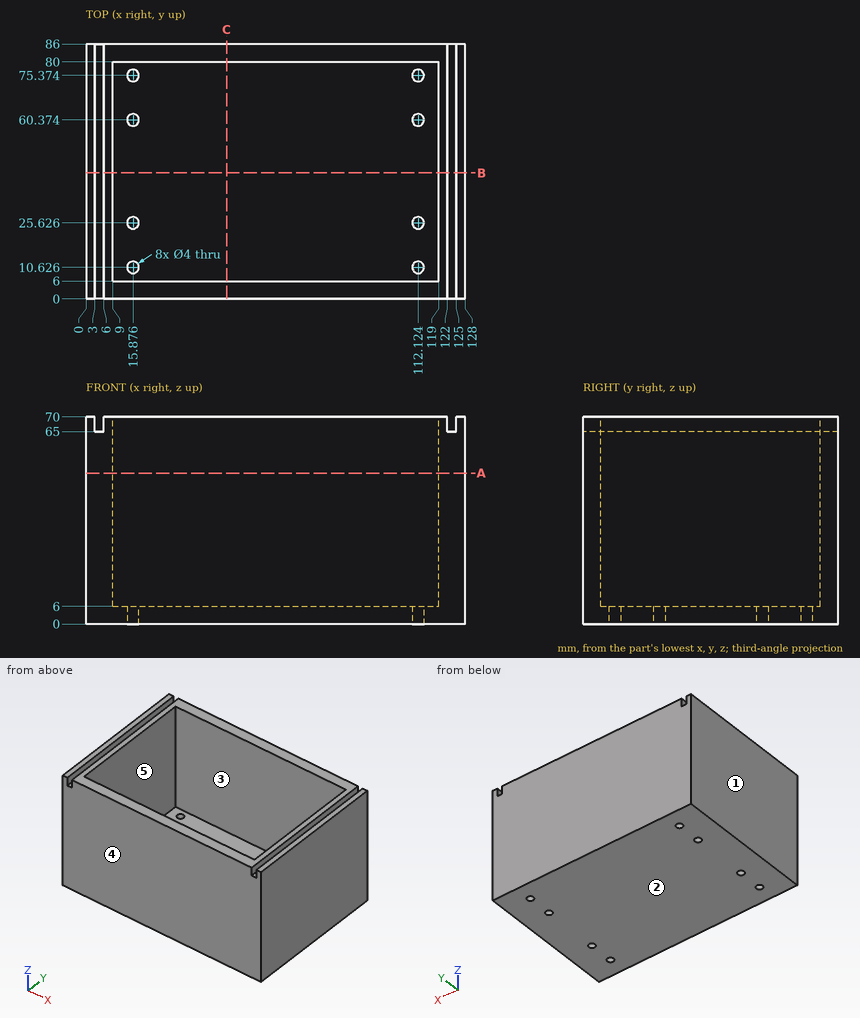
Part print with two shaded views. Sizes in mm from the minimum x, y, z corner. A direction names the side the tool comes from. Coordinates: 2 decimals unless noted, no trailing zeros. Write each loop counter-clockwise with the first axis right and the second up, starting at its lowest first coordinate (ties: lowest second). Pieces come first, ordered by that corner, then holes. Notation, with made-up numbers: (-27, -26) - (-6, -26) arc R19 ccw to (-6, -13) - close; hole circle Ø3 at (-12, -20.5). An arc over 180 degrees is marked (long way). One line per item, written item: value. Start each with the question number.
1. Slice it at B-B (y = 42.5). Write the cut outline in (x, z), plus the area to 3 significant figures.
2. Tool access for the marked faces 4 and 5: list every direction of +Z, -Z, +X, -X, +Y, -Y with a clear straight run to the whole face (end or side of a thin tool).
3. Slice it at C-C (x = 47.5). Write the cut outline in (y, z).
4. Probe line 1 (Y direction, x = 75, z = 52.5); line 2 (X direction, y = 79.5, z = 45.5); line 3 (Z direction, x = 44.5, y = 78.5). List the from-to ranges inside material, lowest first. Write a range as from..to.
5. Slice it at A-A (z = 51). Write the cut outline in (x, y).
6. Flat gauge pins, fed straight in: pin 1 (1 mm diameter, centred on x = 24, y = 16, fed in from +Z); pin 2 (6 mm diameter, centred on x = 19.5, y = 15.5, fed in from -Z); pin 3 (0.9 mm diameter, centred on x = 124, y = 52.5, fed in from +Z); pin 4 (2.5 mm diameter, centred on x = 112.12, y = 10.63, fed in from -Z). Where does each tip first touch, or does it go through?
7. Mould opens along X. For the marked faces 1, 2 and 3 say: released by +X, released by -X, zero draft, split by the parting line, or undercut.
Answers below:
1. outline: (0, 0) - (128, 0) - (128, 70) - (125, 70) - (125, 65) - (122, 65) - (122, 70) - (119, 70) - (119, 6) - (9, 6) - (9, 70) - (6, 70) - (6, 65) - (3, 65) - (3, 70) - (0, 70) - close
1. area: 1,890 mm^2
2. face 4: +Z, -Z, +X, -X, -Y
2. face 5: +Z
3. outline: (0, 0) - (86, 0) - (86, 70) - (80, 70) - (80, 6) - (6, 6) - (6, 70) - (0, 70) - close
4. line 1: y = 0..6, 80..86
4. line 2: x = 0..9, 119..128
4. line 3: z = 0..6
5. outline: (0, 0) - (128, 0) - (128, 86) - (0, 86) - close; hole (9, 6) - (119, 6) - (119, 80) - (9, 80) - close
6. pin 1: stops at z = 6
6. pin 2: stops at z = 0
6. pin 3: stops at z = 65
6. pin 4: passes through
7. face 1: released by -X
7. face 2: zero draft
7. face 3: undercut
